The model under review builds one solid part; all positions refer to its coordinate system, in mm. Round coordinates to 2 decimals unless told otherwise and drop trailing zeros. One line per item, written item: value. Start each with the question number.
from build123d import *

# Parameters (mm, degrees)
F0_W      = 151.1122360826
F0_H      = 52.3923374712
F0_R      = 3.8560302153
F2_DEPTH  = 508
F3_DEPTH  = 25.4
F2_FACE_W = 151.1122360826
F2_FACE_H = 52.3923374712
F2_FACE_R = 3.8560302153
F4_DEPTH  = 25.4


# Not quite as in the source:
# - the program builds the solid bodies; features that only make, move or delete a surface that nothing else refers to are left out


with BuildPart() as f2:
    # F0 (on Right) → F2 (new body)
    with BuildSketch(Plane.YZ):
        with Locations((-0.8284635842, 35.1436007768)):
            Rectangle(F0_W, F0_H)
        with Locations((-69.7291195393, 14.2931053415)):
            Circle(F0_R, mode=Mode.SUBTRACT)
        with Locations((-59.2672452331, 14.7290164605)):
            Circle(F0_R, mode=Mode.SUBTRACT)
        with Locations((-41.3948856294, 14.511060901)):
            Circle(F0_R, mode=Mode.SUBTRACT)
        with Locations((-70.3829824924, 28.2422658056)):
            Circle(F0_R, mode=Mode.SUBTRACT)
        with Locations((-59.0492933989, 27.8063565493)):
            Circle(F0_R, mode=Mode.SUBTRACT)
        with Locations((-49.6772006154, 17.7803952247)):
            Circle(F0_R, mode=Mode.SUBTRACT)
        with Locations((-41.6128411889, 28.8961324841)):
            Circle(F0_R, mode=Mode.SUBTRACT)
        with Locations((-8.7015386671, 15.6008386984)):
            Circle(F0_R, mode=Mode.SUBTRACT)
        with Locations((-33.7664373219, 22.3574638367)):
            Circle(F0_R, mode=Mode.SUBTRACT)
        with Locations((-22.432744503, 17.7803952247)):
            Circle(F0_R, mode=Mode.SUBTRACT)
        with Locations((-24.6123000979, 28.4602232277)):
            Circle(F0_R, mode=Mode.SUBTRACT)
        with Locations((-12.6247387379, 25.6267972291)):
            Circle(F0_R, mode=Mode.SUBTRACT)
        with Locations((-67.5495639443, 39.3580049276)):
            Circle(F0_R, mode=Mode.SUBTRACT)
        with Locations((-58.1774711609, 39.3580049276)):
            Circle(F0_R, mode=Mode.SUBTRACT)
        with Locations((-48.8053783774, 43.2812049985)):
            Circle(F0_R, mode=Mode.SUBTRACT)
        with Locations((-61.0108934343, 49.6019162238)):
            Circle(F0_R, mode=Mode.SUBTRACT)
        with Locations((-69.9470713735, 55.7046793401)):
            Circle(F0_R, mode=Mode.SUBTRACT)
        with Locations((-52.7285784483, 53.7430755794)):
            Circle(F0_R, mode=Mode.SUBTRACT)
        with Locations((-39.2153263092, 53.9610348642)):
            Circle(F0_R, mode=Mode.SUBTRACT)
        with Locations((-30.7150576264, 36.3066233695)):
            Circle(F0_R, mode=Mode.SUBTRACT)
        with Locations((-37.6896373928, 43.499160558)):
            Circle(F0_R, mode=Mode.SUBTRACT)
        with Locations((-20.4711426049, 44.8068939149)):
            Circle(F0_R, mode=Mode.SUBTRACT)
        with Locations((-13.9324739575, 37.6143604517)):
            Circle(F0_R, mode=Mode.SUBTRACT)
        with Locations((-6.9578932598, 41.9734716415)):
            Circle(F0_R, mode=Mode.SUBTRACT)
        with Locations((-28.5355020314, 46.5505383909)):
            Circle(F0_R, mode=Mode.SUBTRACT)
        with Locations((-23.0866111815, 55.7046793401)):
            Circle(F0_R, mode=Mode.SUBTRACT)
        with Locations((-11.0990498215, 50.6916977465)):
            Circle(F0_R, mode=Mode.SUBTRACT)
        with Locations((14.83767014, 15.1649275795)):
            Circle(F0_R, mode=Mode.SUBTRACT)
        with Locations((29.8766102642, 14.2931053415)):
            Circle(F0_R, mode=Mode.SUBTRACT)
        with Locations((2.8501115739, 19.9599526823)):
            Circle(F0_R, mode=Mode.SUBTRACT)
        with Locations((3.5039787181, 29.767954722)):
            Circle(F0_R, mode=Mode.SUBTRACT)
        with Locations((11.5683367476, 28.0243102461)):
            Circle(F0_R, mode=Mode.SUBTRACT)
        with Locations((21.8122527003, 26.9345343113)):
            Circle(F0_R, mode=Mode.SUBTRACT)
        with Locations((38.5948345065, 23.2292860746)):
            Circle(F0_R, mode=Mode.SUBTRACT)
        with Locations((46.659193933, 18.8701730222)):
            Circle(F0_R, mode=Mode.SUBTRACT)
        with Locations((51.2362644076, 30.6397788227)):
            Circle(F0_R, mode=Mode.SUBTRACT)
        with Locations((59.0826645494, 19.7419971228)):
            Circle(F0_R, mode=Mode.SUBTRACT)
        with Locations((68.0188462138, 17.5624396652)):
            Circle(F0_R, mode=Mode.SUBTRACT)
        with Locations((67.8008943796, 31.0756899416)):
            Circle(F0_R, mode=Mode.SUBTRACT)
        with Locations((3.5039787181, 40.0118716061)):
            Circle(F0_R, mode=Mode.SUBTRACT)
        with Locations((13.0940265954, 43.499160558)):
            Circle(F0_R, mode=Mode.SUBTRACT)
        with Locations((35.1075492799, 37.3964048922)):
            Circle(F0_R, mode=Mode.SUBTRACT)
        with Locations((22.0302101225, 41.3196049631)):
            Circle(F0_R, mode=Mode.SUBTRACT)
        with Locations((3.2860212959, 49.8198717833)):
            Circle(F0_R, mode=Mode.SUBTRACT)
        with Locations((14.1838034615, 54.6148978174)):
            Circle(F0_R, mode=Mode.SUBTRACT)
        with Locations((26.3893213123, 51.5635199845)):
            Circle(F0_R, mode=Mode.SUBTRACT)
        with Locations((35.5434566736, 49.8198717833)):
            Circle(F0_R, mode=Mode.SUBTRACT)
        with Locations((43.8257716596, 38.4861826897)):
            Circle(F0_R, mode=Mode.SUBTRACT)
        with Locations((51.0183051229, 44.3709865212)):
            Circle(F0_R, mode=Mode.SUBTRACT)
        with Locations((59.0826645494, 38.2682271302)):
            Circle(F0_R, mode=Mode.SUBTRACT)
        with Locations((46.659193933, 55.0508089364)):
            Circle(F0_R, mode=Mode.SUBTRACT)
        with Locations((66.2752017379, 46.5505383909)):
            Circle(F0_R, mode=Mode.SUBTRACT)
        with Locations((59.5185756683, 54.6148978174)):
            Circle(F0_R, mode=Mode.SUBTRACT)
        with Locations((-69.9470713735, 55.7046793401)):
            Circle(F0_R)
    extrude(amount=F2_DEPTH)

    # F0 (on Right) → F3 (join)
    with BuildSketch(Plane.YZ):
        with Locations((-61.0108934343, 49.6019162238)):
            Circle(F0_R)
    extrude(amount=F3_DEPTH)

    # F2_face (on face) + F0 (on Right) → F4 (join)
    with BuildSketch(Plane(origin=(508, -0.362148073, 35.2651590305), x_dir=(0, 1, 0), z_dir=(1, 0, 0))):
        with Locations((-0.4663155112, -0.1215582537)):
            Rectangle(F2_FACE_W, F2_FACE_H)
        with Locations((-69.3669714662, -20.972053689)):
            Circle(F2_FACE_R, mode=Mode.SUBTRACT)
        with Locations((-58.90509716, -20.53614257)):
            Circle(F2_FACE_R, mode=Mode.SUBTRACT)
        with Locations((-41.0327375564, -20.7540981295)):
            Circle(F2_FACE_R, mode=Mode.SUBTRACT)
        with Locations((-70.0208344194, -7.0228932249)):
            Circle(F2_FACE_R, mode=Mode.SUBTRACT)
        with Locations((-58.6871453258, -7.4588024812)):
            Circle(F2_FACE_R, mode=Mode.SUBTRACT)
        with Locations((-49.3150525424, -17.4847638058)):
            Circle(F2_FACE_R, mode=Mode.SUBTRACT)
        with Locations((-41.2506931159, -6.3690265464)):
            Circle(F2_FACE_R, mode=Mode.SUBTRACT)
        with Locations((-8.3393905941, -19.664320332)):
            Circle(F2_FACE_R, mode=Mode.SUBTRACT)
        with Locations((-33.4042892489, -12.9076951938)):
            Circle(F2_FACE_R, mode=Mode.SUBTRACT)
        with Locations((-22.07059643, -17.4847638058)):
            Circle(F2_FACE_R, mode=Mode.SUBTRACT)
        with Locations((-24.2501520249, -6.8049358027)):
            Circle(F2_FACE_R, mode=Mode.SUBTRACT)
        with Locations((-12.2625906649, -9.6383618014)):
            Circle(F2_FACE_R, mode=Mode.SUBTRACT)
        with Locations((-67.1874158713, 4.0928458972)):
            Circle(F2_FACE_R, mode=Mode.SUBTRACT)
        with Locations((-57.8153230879, 4.0928458972)):
            Circle(F2_FACE_R, mode=Mode.SUBTRACT)
        with Locations((-48.4432303044, 8.016045968)):
            Circle(F2_FACE_R, mode=Mode.SUBTRACT)
        with Locations((-60.6487453613, 14.3367571933)):
            Circle(F2_FACE_R, mode=Mode.SUBTRACT)
        with Locations((59.8807237414, 19.3497387869)):
            Circle(F2_FACE_R, mode=Mode.SUBTRACT)
        with Locations((-52.3664303753, 18.4779165489)):
            Circle(F2_FACE_R, mode=Mode.SUBTRACT)
        with Locations((-38.8531782362, 18.6958758337)):
            Circle(F2_FACE_R, mode=Mode.SUBTRACT)
        with Locations((-30.3529095533, 1.041464339)):
            Circle(F2_FACE_R, mode=Mode.SUBTRACT)
        with Locations((-37.3274893197, 8.2340015275)):
            Circle(F2_FACE_R, mode=Mode.SUBTRACT)
        with Locations((-20.1089945319, 9.5417348845)):
            Circle(F2_FACE_R, mode=Mode.SUBTRACT)
        with Locations((-13.5703258845, 2.3492014212)):
            Circle(F2_FACE_R, mode=Mode.SUBTRACT)
        with Locations((-6.5957451868, 6.7083126111)):
            Circle(F2_FACE_R, mode=Mode.SUBTRACT)
        with Locations((-28.1733539584, 11.2853793604)):
            Circle(F2_FACE_R, mode=Mode.SUBTRACT)
        with Locations((-22.7244631085, 20.4395203097)):
            Circle(F2_FACE_R, mode=Mode.SUBTRACT)
        with Locations((-10.7369017485, 15.4265387161)):
            Circle(F2_FACE_R, mode=Mode.SUBTRACT)
        with Locations((15.199818213, -20.100231451)):
            Circle(F2_FACE_R, mode=Mode.SUBTRACT)
        with Locations((30.2387583372, -20.972053689)):
            Circle(F2_FACE_R, mode=Mode.SUBTRACT)
        with Locations((3.212259647, -15.3052063482)):
            Circle(F2_FACE_R, mode=Mode.SUBTRACT)
        with Locations((3.8661267911, -5.4972043084)):
            Circle(F2_FACE_R, mode=Mode.SUBTRACT)
        with Locations((11.9304848206, -7.2408487843)):
            Circle(F2_FACE_R, mode=Mode.SUBTRACT)
        with Locations((22.1744007734, -8.3306247192)):
            Circle(F2_FACE_R, mode=Mode.SUBTRACT)
        with Locations((38.9569825795, -12.0358729558)):
            Circle(F2_FACE_R, mode=Mode.SUBTRACT)
        with Locations((47.021342006, -16.3949860083)):
            Circle(F2_FACE_R, mode=Mode.SUBTRACT)
        with Locations((51.5984124807, -4.6253802078)):
            Circle(F2_FACE_R, mode=Mode.SUBTRACT)
        with Locations((59.4448126224, -15.5231619077)):
            Circle(F2_FACE_R, mode=Mode.SUBTRACT)
        with Locations((68.3809942868, -17.7027193653)):
            Circle(F2_FACE_R, mode=Mode.SUBTRACT)
        with Locations((68.1630424526, -4.1894690888)):
            Circle(F2_FACE_R, mode=Mode.SUBTRACT)
        with Locations((3.8661267911, 4.7467125757)):
            Circle(F2_FACE_R, mode=Mode.SUBTRACT)
        with Locations((13.4561746684, 8.2340015275)):
            Circle(F2_FACE_R, mode=Mode.SUBTRACT)
        with Locations((35.469697353, 2.1312458618)):
            Circle(F2_FACE_R, mode=Mode.SUBTRACT)
        with Locations((22.3923581955, 6.0544459326)):
            Circle(F2_FACE_R, mode=Mode.SUBTRACT)
        with Locations((3.648169369, 14.5547127528)):
            Circle(F2_FACE_R, mode=Mode.SUBTRACT)
        with Locations((14.5459515345, 19.3497387869)):
            Circle(F2_FACE_R, mode=Mode.SUBTRACT)
        with Locations((26.7514693853, 16.298360954)):
            Circle(F2_FACE_R, mode=Mode.SUBTRACT)
        with Locations((35.9056047466, 14.5547127528)):
            Circle(F2_FACE_R, mode=Mode.SUBTRACT)
        with Locations((44.1879197326, 3.2210236592)):
            Circle(F2_FACE_R, mode=Mode.SUBTRACT)
        with Locations((51.3804531959, 9.1058274908)):
            Circle(F2_FACE_R, mode=Mode.SUBTRACT)
        with Locations((59.4448126224, 3.0030680997)):
            Circle(F2_FACE_R, mode=Mode.SUBTRACT)
        with Locations((47.021342006, 19.7856499059)):
            Circle(F2_FACE_R, mode=Mode.SUBTRACT)
        with Locations((66.6373498109, 11.2853793604)):
            Circle(F2_FACE_R, mode=Mode.SUBTRACT)
    with BuildSketch(Plane.YZ):
        with Locations((-41.6128411889, 28.8961324841)):
            Circle(F0_R)
        with Locations((-37.6896373928, 43.499160558)):
            Circle(F0_R)
        with Locations((-24.6123000979, 28.4602232277)):
            Circle(F0_R)
        with Locations((38.5948345065, 23.2292860746)):
            Circle(F0_R)
    extrude(amount=F4_DEPTH)


solid = f2.part
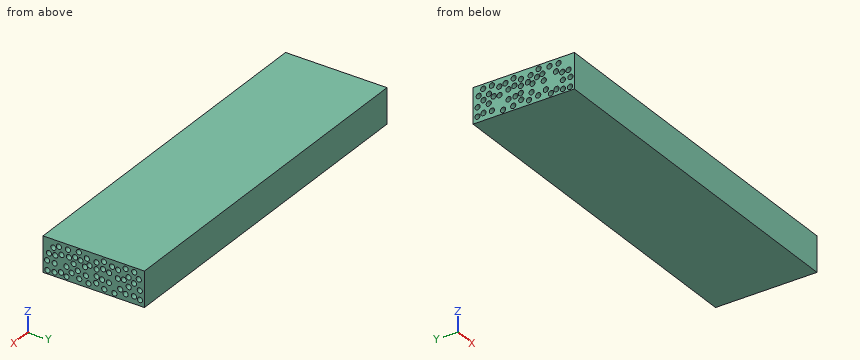
Item 1: Clearance check with a flat-ended pin moving along its axis: P1, Ø6, axis at y = 59.52, z = 54.61, coming from the -X side. State where the tip first meets the part, or that it passes through.
Item 2: Consider section A-A, the plane x = 168. Count the separate pieces of the cut face and the enclosed holes in it, then the cut area to 3 significant figures.
Item 3: Wall thickness on L1, parallel to Z at x = 37.5, y = -28; L2, parallel to Z at x = 153.5, y = -32; L3, parallel to Z at x = 87, y = 34.5: over which ranges is each line inside the solid? List them lowest first.
Computed:
1. P1: passes through
2. separate pieces: 1
2. enclosed holes: 52
2. area: 5,490 mm^2
3. L1: z = 8.95 to 26.62, 30.3 to 33.57, 39.04 to 42.73, 50.37 to 61.34
3. L2: z = 8.95 to 18.93, 25.79 to 32.67, 39.94 to 44.86, 48.24 to 61.34
3. L3: z = 8.95 to 33.59, 41.2 to 46.11, 53.53 to 61.34
